Build history of the part. All positions in model axes, mm. A direction names the side the tool comes from. Coordinates: 2 decimals unless noted, no trailing zeros. Order: outer loops, then holes, each group sorted by start corner. A loop starts at its lowest first (then second) coordinate and runs counter-clockwise, first axis right, second up. Notation, with made-up numbers: (77, -13.5) - (103, -13.5) arc R21 ccw to (103, -2.5) - close; hole circle Ø5 at (-12.75, 22.5). An arc over 180 degrees is marked (long way). Answer as CSV lines item,"result". Start each with the question number.
from build123d import *

# Parameters (mm, degrees)
SKETCH_1_W                   = 300
SKETCH_1_H                   = 15
EXTRUDE_349_DEPTH            = 15
HOLE_WIZARD_M6_D             = 5
HOLE_WIZARD_M6_CSINK_D       = 12.6
HOLE_WIZARD_M6_CSINK_ANGLE   = 90
HOLE_WIZARD_M8_D             = 6.8
SKETCH_8_W                   = 250
SKETCH_8_H                   = 15
EXTRUDE_2463_DEPTH           = 5.4
SKETCH_9_R                   = 4
CUT_EXTRUDE_2783_DEPTH       = 1.5
SKETCH_10_W                  = 100
SKETCH_10_H                  = 15
CUT_EXTRUDE_3071_DEPTH       = 5.4
HOLE_WIZARD_1_M6_D           = 5
HOLE_WIZARD_1_M6_CSINK_D     = 12.6
HOLE_WIZARD_1_M6_CSINK_ANGLE = 90
HOLE_WIZARD_2_M6_D           = 5
HOLE_WIZARD_2_M6_CSINK_D     = 12.6
HOLE_WIZARD_2_M6_CSINK_ANGLE = 90
FILLET_1_R                   = 3
CHAMFER_1_SIZE               = 5
CHAMFER_2_SIZE               = 1


with BuildPart() as part:
    # Эскиз1 → Extrude 349 (new body)
    with BuildSketch(Plane(origin=(0, 0, 0), x_dir=(1, 0, 0), z_dir=(0, 1, 0))):
        Rectangle(SKETCH_1_W, SKETCH_1_H)
    extrude(amount=EXTRUDE_349_DEPTH)

    # Крепление шарнира M6 (through all)
    with Locations(Plane(origin=(0, 15, 0), x_dir=(1, 0, 0), z_dir=(0, 1, 0))):
        with Locations((-115, 0), (115, 0)):
            CounterSinkHole(HOLE_WIZARD_M6_D / 2, HOLE_WIZARD_M6_CSINK_D / 2, counter_sink_angle=HOLE_WIZARD_M6_CSINK_ANGLE)

    # Шпилька-M8 (through all)
    with Locations(Plane(origin=(0, 15, 0), x_dir=(1, 0, 0), z_dir=(0, 1, 0))):
        with Locations((-140, 0), (140, 0)):
            Hole(HOLE_WIZARD_M8_D / 2)

    # Эскиз8 → Extrude 2463 (add)
    with BuildSketch(Plane.XY.offset(7.5)):
        with Locations((0, 7.5)):
            Rectangle(SKETCH_8_W, SKETCH_8_H)
    extrude(amount=EXTRUDE_2463_DEPTH)

    # Эскиз9 → Cut-Extrude 2783 (cut)
    with BuildSketch(Plane.XY.offset(12.9)):
        with Locations((-105, 7.5)):
            Circle(SKETCH_9_R)
        with Locations((105, 7.5)):
            Circle(SKETCH_9_R)
    extrude(amount=-CUT_EXTRUDE_2783_DEPTH, mode=Mode.SUBTRACT)

    # Эскиз10 → Cut-Extrude 3071 (cut)
    with BuildSketch(Plane.XY.offset(12.9)):
        with Locations((0, 7.5)):
            Rectangle(SKETCH_10_W, SKETCH_10_H)
    extrude(amount=-CUT_EXTRUDE_3071_DEPTH, mode=Mode.SUBTRACT)

    # Прижим-1-M6 (through all)
    with Locations(Plane.XY.offset(12.9)):
        with Locations((-90, 7.5), (90, 7.5)):
            CounterSinkHole(HOLE_WIZARD_1_M6_D / 2, HOLE_WIZARD_1_M6_CSINK_D / 2, counter_sink_angle=HOLE_WIZARD_1_M6_CSINK_ANGLE)

    # Прижим-2-M6 (through all)
    with Locations(Plane.XY.offset(7.5)):
        with Locations((-30, 7.5), (30, 7.5)):
            CounterSinkHole(HOLE_WIZARD_2_M6_D / 2, HOLE_WIZARD_2_M6_CSINK_D / 2, counter_sink_angle=HOLE_WIZARD_2_M6_CSINK_ANGLE)

    # Скругление1
    fillet_1_edges = [part.edges().sort_by_distance(p)[0] for p in [
        (-50, 0, 10.2),
        (50, 0, 10.2),
    ]]
    fillet(fillet_1_edges, radius=FILLET_1_R)

    # Фаска1
    chamfer_1_edges = [part.edges().sort_by_distance(p)[0] for p in [
        (-150, 7.5, -7.5),
        (150, 7.5, -7.5),
    ]]
    chamfer(chamfer_1_edges, length=CHAMFER_1_SIZE)

    # Фаска2
    chamfer_2_edges = [part.edges().sort_by_distance(p)[0] for p in [
        (-50.878679656, 0.878679656, 12.9),
        (-125, 7.5, 12.9),
        (-89, 0, 12.9),
        (125, 7.5, 12.9),
        (-50, 9, 12.9),
        (50, 9, 12.9),
        (89, 0, 12.9),
        (50.878679656, 0.878679656, 12.9),
    ]]
    chamfer(chamfer_2_edges, length=CHAMFER_2_SIZE)


solid = part.part
(1) Drop flat-ended pins along their axis: pin 1 Ø4.5 at (x, y) = (6, 5.5) entering from +Z; pin 2 Ø1.3 at (y, z) = (8, 11) entering from +X; pin 3 Ø3.5 at (y, z) = (7, 10) entering from -X. Give the stop position or say it passes through.
(2) Band-saw the part on D-D on x = 105. List the corners of the cut face in (y, z), plus the area to 4 significant figures.
(3) Band-saw the part on A-A on z = 0. State how many separate pieces and enclosed holes the cut face has, plus the area to 3 significant figures.
(4) Band-saw the part on B-B on x = 30. List the corners of the cut face in (y, z).
(5) Probe L1, parallel to Y at x = -30, z = -2; L2, parallel to Z at x = 140, y = 10.5; L3, parallel to Z at x = -41, y = 2.25. List the from-to ranges inside material, lowest first. Write a range as [from, to].
(6) Pull direction Z, two halves, no side cores. Call faces 1 (the cylindrical face through (92, 6, 1)), 2 (the flat face through (-1, 8, 7.5)), 3 (the conical face through (117.7, 11.4, -0.1)): +Z half, -Z half, draft (parallel to the pull), parting line (faces both ways), or undercut.
(7) Which spindle directions (+Z, -Z, +X, -X, +Y, -Y) get a long thin tool onto all of the face, cutting with end or side? Do faces 4 (the flat face through (-105, 8, 11.4)), 5 (the flat face through (137, 7, 7.5)), 6 (the cylindrical face through (-88, 6, 1)). Say none if no direction does.
Filled in:
1,pin 1,"stops at z = 7.5"
1,pin 2,"stops at x = 125"
1,pin 3,"stops at x = -125"
2,outline,"(0, -7.5) - (15, -7.5) - (15, 12.9) - (11.5, 12.9) - (11.5, 11.4) - (3.5, 11.4) - (3.5, 12.9) - (1, 12.9) - (0, 11.9) - close"
2,area,"293.5 mm^2"
3,separate pieces,"5"
3,enclosed holes,"4"
3,area,"4,040 mm^2"
4,outline,"(0, -7.5) - (5, -7.5) - (5, 3.7) - (1.2, 7.5) - (0, 7.5) - close; (10, -7.5) - (15, -7.5) - (15, 7.5) - (13.8, 7.5) - (10, 3.7) - close"
5,L1,"y = [0, 5], [10, 15]"
5,L2,"z = [-7.5, -3.4], [3.4, 7.5]"
5,L3,"z = [-7.5, 7.5]"
6,face 1,"draft"
6,face 2,"+Z half"
6,face 3,"undercut"
7,face 4,"+Z"
7,face 5,"+Z, +X, +Y, -Y"
7,face 6,"+Z, -Z"
